The figure shows three views and two pictorial views of one solid part (mm, origin at its lowest corner). Answer the questions. Round coordinates to 2 decimals unless told otherwise and drop trailing zeros. Order: outer loops, then holes, each group sorted by start corner. A loop starts at its lowest first (then second) coordinate and runs counter-clockwise, first axis right, second up. Notation, with made-up numbers: (44, 78) - (86, 78) arc R17 cw to (86, 106) - close; hole circle Ø6 at (-40, 5.25). An arc over 180 degrees is marked (long way). Answer as a JSON object with one key per item and string values. Group by question number.
Q1. A cutting plane is placed at C-C on y = 15. Determine the outline of the cut face in (x, z), and give its area (3 significant figures).
Q2. A cutting plane is placed at B-B on z = 4.25. Determine the outline of the cut face in (x, y).
Q3. A cutting plane is placed at A-A on x = 24.5. Determine the outline of the cut face in (y, z), and give its area (4 significant figures).
Q4. Consider line 1 (X direction, y = 74.5, z = 0.4); line 2 (Y direction, x = 36, z = 3.3); line 3 (Y direction, x = 33, z = 0.4). Determine where each line is inside the solid, lowest interval first.
Q5. A cutting plane is placed at D-D on x = 46.5. Determine the outline of the cut face in (y, z), and give its area (3 significant figures).
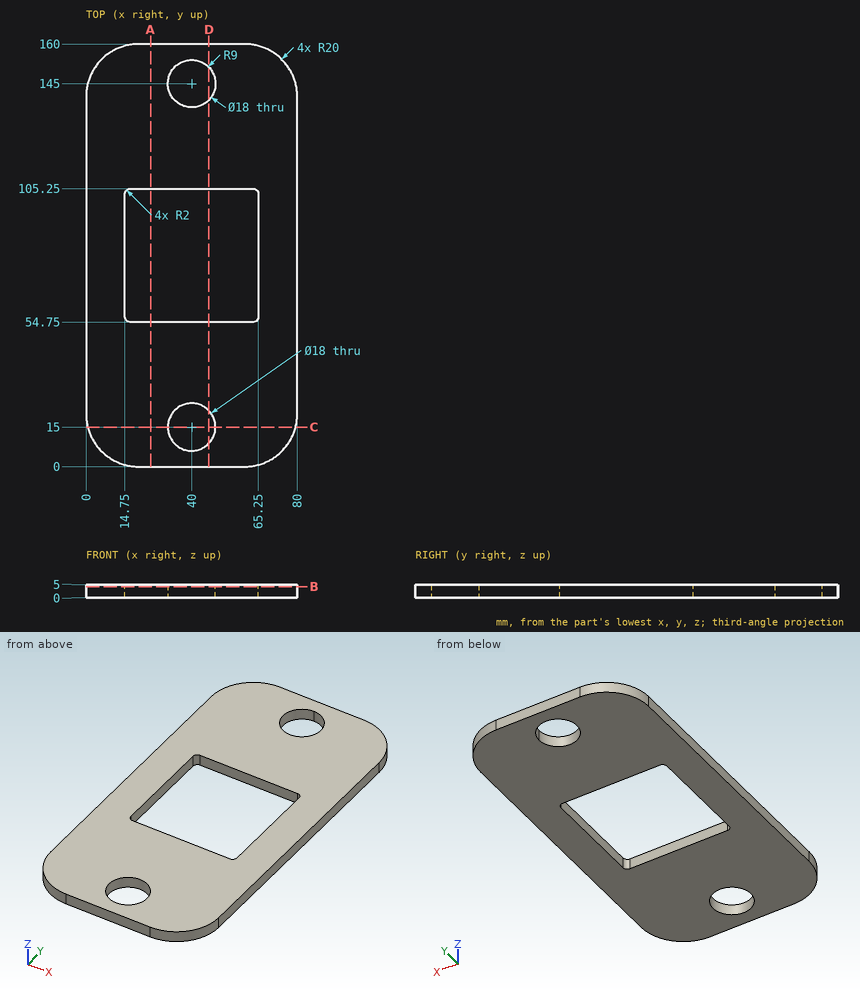
Result set:
{
 "1": {"outline": "(0.64, 0) - (31, 0) - (31, 5) - (0.64, 5) - close; (49, 0) - (79.36, 0) - (79.36, 5) - (49, 5) - close", "area": "304 mm²"},
 "2": {"outline": "(0, 20) arc R20 ccw to (20, 0) - (60, 0) arc R20 ccw to (80, 20) - (80, 140) arc R20 ccw to (60, 160) - (20, 160) arc R20 ccw to (0, 140) - close; hole (14.75, 56.75) arc R2 ccw to (16.75, 54.75) - (63.25, 54.75) arc R2 ccw to (65.25, 56.75) - (65.25, 103.25) arc R2 ccw to (63.25, 105.25) - (16.75, 105.25) arc R2 ccw to (14.75, 103.25) - close; hole circle Ø18 at (40, 15); hole circle Ø18 at (40, 145)"},
 "3": {"outline": "(0, 0) - (54.75, 0) - (54.75, 5) - (0, 5) - close; (105.25, 0) - (160, 0) - (160, 5) - (105.25, 5) - close", "area": "547.5 mm²"},
 "4": {"line 1": "x = 0 to 14.75, 65.25 to 80", "line 2": "y = 0 to 6.94, 23.06 to 54.75, 105.25 to 136.94, 153.06 to 160", "line 3": "y = 0 to 9.34, 20.66 to 54.75, 105.25 to 139.34, 150.66 to 160"},
 "5": {"outline": "(0, 0) - (8.78, 0) - (8.78, 5) - (0, 5) - close; (21.22, 0) - (54.75, 0) - (54.75, 5) - (21.22, 5) - close; (105.25, 0) - (138.78, 0) - (138.78, 5) - (105.25, 5) - close; (151.22, 0) - (160, 0) - (160, 5) - (151.22, 5) - close", "area": "423 mm²"}
}
